from build123d import *

# Parameters (mm, degrees)
BOSS_EXTRU_1_DEPTH      = 55
ESQUISSE2_W             = 36.5
ESQUISSE2_H             = 47
ENL_V_MAT_EXTRU_1_DEPTH = 65.730209331
ESQUISSE3_W             = 5.5
ESQUISSE3_H             = 8
ENL_V_MAT_EXTRU_2_DEPTH = 3
ESQUISSE4_R             = 5.5
ENL_V_MAT_EXTRU_3_DEPTH = 3


with BuildPart() as part:
    # Esquisse1 → Boss.-Extru.1 (new body)
    with BuildSketch(Plane(origin=(0, 0, 0), x_dir=(1, 0, 0), z_dir=(0, 1, 0))):
        Polygon((34, -2.5), (29, 2.5), (18.5, 2.5), (18.5, -0.5), (-26, -0.5), (-26, -2.5), align=None)
    extrude(amount=BOSS_EXTRU_1_DEPTH)

    # Esquisse2 → Enlèv. mat.-Extru.1 (cut, through all)
    with BuildSketch(Plane(origin=(0, 0, 0.5), x_dir=(-1, 0, 0), z_dir=(0, 0, -1))):
        with Locations((-0.25, 23.5)):
            Rectangle(ESQUISSE2_W, ESQUISSE2_H)
    extrude(amount=-ENL_V_MAT_EXTRU_1_DEPTH, mode=Mode.SUBTRACT)

    # Esquisse3 → Enlèv. mat.-Extru.2 (cut)
    with BuildSketch(Plane(origin=(0, 0, -2.5), x_dir=(-1, 0, 0), z_dir=(0, 0, -1))):
        with Locations((-21.25, 51)):
            Rectangle(ESQUISSE3_W, ESQUISSE3_H)
    extrude(amount=-ENL_V_MAT_EXTRU_2_DEPTH, mode=Mode.SUBTRACT)

    # Esquisse4 → Enlèv. mat.-Extru.3 (cut)
    with BuildSketch(Plane.XZ):
        with Locations((29, 2.5)):
            Circle(ESQUISSE4_R)
    extrude(amount=-ENL_V_MAT_EXTRU_3_DEPTH, mode=Mode.SUBTRACT)


solid = part.part
Input: part model. Units: mm. Frame: model coordinates. A direction names the side the tool comes from. Coordinates: 2 decimals unless noted, no trailing zeros. Loops run counter-clockwise (first coordinate to the right, second up) from the corner with the lowest first, then second, coordinate; pieces in that order, holes last.
(1) Section A-A on y = 18. Return the cut outline in (x, z), then the cut area to 3 significant figures.
(2) Set-up query: faces 1 (the face through (-22, 0, 1)), 2 (the face through (28, 3, 1)), 3 (the face through (1, 47, 1)), 4 (the face through (24, 51, -1)), 5 (the face through (31.5, 28.6, 0)). Return all of +Z, -Z, +X, -X, +Y, -Y with unobstructed straight access to the full face (end or side cutting, diameter ignored); none if empty.
(3) Section B-B on x = 22. Return the cut outline in (y, z).
(4) Material intervals for probe 1 along X at (y, z) = (22.5, 0.6); probe 2 along Z at (x, y) = (-4.5, 52); probe 3 along Y at (x, z) = (22, 0), sorted ascending.
(5) Section C-C on z = -1.4. Return the cut outline in (x, y), then the cut area to 3 significant figures.
(6) Section D-D on y = 48. Return the cut outline in (x, z).
(7) First-contact query: pin 1 Ø2 at (y, z) = (19.5, 2) entering from +X; pin 2 Ø2.5 at (x, z) = (28, 0.5) entering from -Y; pin 3 Ø1.6 at (x, z) = (1.5, 1.5) entering from -Y; pin 4 Ø25 at (x, y) = (1, 25) entering from -Z. Flat tips, straight axial feed; report the tip coordinate or a pass-through.
(8) Pull-direction query (X, two-part tool) for faces 6 (the face through (24, 33, 2.5)), 7 (the face through (-18, 23, 1)), 8 (the face through (-26, 27, 1)); classes: released by +X, released by -X, zero draft, split by the parting line, or undercut.
Data:
1. outline: (-26, 0.5) - (-18, 0.5) - (-18, 2.5) - (-26, 2.5) - close; (18.5, -2.5) - (29, -2.5) - (34, 2.5) - (18.5, 2.5) - close
1. area: 81.0 mm2
2. face 1: +Z, -Z, +X, -X, -Y
2. face 2: +Z, +X, -Y
2. face 3: +Z, -Z, -Y
2. face 4: -Z, -X, +Y
2. face 5: -Z, +X, +Y, -Y
3. outline: (0, -2.5) - (47, -2.5) - (47, 0.5) - (55, 0.5) - (55, 2.5) - (0, 2.5) - close
4. probe 1: x = -26 to -18, 18.5 to 32.1
4. probe 2: z = 0.5 to 2.5
4. probe 3: y = 0 to 47
5. outline: (18.5, 0) - (25.12, 0) - (25.12, 3) - (30.1, 3) - (30.1, 55) - (24, 55) - (24, 47) - (18.5, 47) - close
5. area: 579 mm2
6. outline: (-26, 0.5) - (24, 0.5) - (24, -2.5) - (29, -2.5) - (34, 2.5) - (-26, 2.5) - close
7. pin 1: stops at x = 34
7. pin 2: stops at y = 3
7. pin 3: stops at y = 47
7. pin 4: passes through
8. face 6: zero draft
8. face 7: undercut
8. face 8: released by -X
